```python
from build123d import *

# Parameters (mm, degrees)
F0_W     = 225.6237479062
F0_H     = 127
F0_R     = 25.7058012272
F1_DEPTH = 94.996
F1_TAPER = -10


with BuildPart() as f1:
    # F0 (on Top) → F1 (new body)
    with BuildSketch(Plane.XY):
        with Locations((23.1080837548, -16.8385943398)):
            Rectangle(F0_W, F0_H)
        with Locations((18.8035357351, -18.2947983858)):
            Circle(F0_R, mode=Mode.SUBTRACT)
    extrude(amount=F1_DEPTH, taper=F1_TAPER)


solid = f1.part
```
The model under review builds one solid part; all positions refer to its coordinate system, in mm. Coordinates: 2 decimals unless noted, no trailing zeros.
1) The part is to be moulded in two halves that separate along X. For faces 1 (the face through (46, -2, 0)), 2 (the face through (28.06, -32.81, 48.16)), say which applies: pulls with the +X half, pulls with the -X half, needs draft (parallel to the pull), parting line crosses it, or undercut.
2) To check wall thickness, follow probe 1 along X at (y, z) = (-2.5, 19); probe 2 along X at (y, z) = (-34.5, 45.5); probe 3 along X at (y, z) = (22.5, 82.5). State the ranges of each line that lie inside material, in increasing order.
3) Clearance check with flat-ended pins moving along their axes: pin 1 Ø3 at (x, z) = (119, 40) entering from +Y; pin 2 Ø2 at (x, y) = (59.5, -40) entering from -Z; pin 3 Ø1 at (y, z) = (-73.5, 48.5) entering from +X; pin 4 Ø3 at (y, z) = (-27, 85) entering from +X. State where each tip first meets the part, or that it passes through.
Answer list:
1. face 1: needs draft
1. face 2: undercut
2. probe 1: x = -93.05 to 2.98, 34.62 to 139.27
2. probe 2: x = -97.73 to 11.73, 25.88 to 143.94
2. probe 3: x = -104.25 to 150.47
3. pin 1: stops at y = 53.98
3. pin 2: stops at z = 0
3. pin 3: stops at x = 144.56
3. pin 4: stops at x = 151.17
